Work out the finished part from the listing and answer in its coordinate system (mm). A direction names the side the tool comes from. Coordinates: 2 decimals unless noted, no trailing zeros. Order: outer loops, then holes, each group sorted by start corner. A loop starts at its lowest first (then second) coordinate and runs counter-clockwise, first axis right, second up. Notation, with made-up numbers: (46, -37.75) - (85, -37.75) arc R27 ccw to (85, -12.75) - close; hole circle Ø9 at (75, -19.5). An arc over 180 degrees is marked (long way). Use CSV: the item, a comma, the result in double quotes. Start each with the question number.
from build123d import *

# Parameters (mm, degrees)
SKETCH1_W           = 12
SKETCH1_H           = 10
BOSS_EXTRUDE1_DEPTH = 24.2
SKETCH2_R           = 1.5
BOSS_EXTRUDE2_DEPTH = 10
SKETCH3_R           = 0.65
CUT_EXTRUDE1_DEPTH  = 1


with BuildPart() as part:
    # Sketch1 → Boss-Extrude1 (new body)
    with BuildSketch(Plane(origin=(0, 0, 0), x_dir=(0, 0, -1), z_dir=(1, 0, 0))):
        Rectangle(SKETCH1_W, SKETCH1_H)
    extrude(amount=BOSS_EXTRUDE1_DEPTH)

    # Sketch2 → Boss-Extrude2 (add)
    with BuildSketch(Plane(origin=(24.2, 0, 0), x_dir=(0, 0, -1), z_dir=(1, 0, 0))):
        Circle(SKETCH2_R)
    extrude(amount=BOSS_EXTRUDE2_DEPTH)

    # Sketch3 → Cut-Extrude1 (cut)
    with BuildSketch(Plane(origin=(24.2, 0, 0), x_dir=(0, 0, -1), z_dir=(1, 0, 0))):
        with Locations((-4.5, 0)):
            Circle(SKETCH3_R)
        with Locations((4.5, 0)):
            Circle(SKETCH3_R)
    extrude(amount=-CUT_EXTRUDE1_DEPTH, mode=Mode.SUBTRACT)


solid = part.part
1) Straight lines are drawn through the part: line 1 (Y direction, x = 23.85, z = -4.5); line 2 (X direction, y = 4.25, z = 3.25). For each, find the intervals that lie inside material, in ascending order. Write a range as [from, to].
2) For faces 1 (the face through (23.71, 0.2, 3.88)), 2 (the face through (12, 0, -6)), determine the directions among +Z, -Z, +X, -X, +Y, -Y from which every point of the face is accessible in a straight line to the end or side of a thin tool.
3) The part is cut by section D-D on y = -3.5. Determine the outline of the cut face in (x, z), plus the area to 3 significant figures.
4) The part is cut by section B-B on y = 0. Determine the outline of the cut face in (x, z).
5) Flat-ended cylindrical pins translate along their axes: P1, Ø2, axis at y = 0, z = -4.5, coming from the +X side; P2, Ø5, axis at y = 1, z = 2, coming from the +X side. Find the tip coordinate at first contact, or state that the pin passes through.
6) The part is cut by section C-C on z = -4.5. Determine the outline of the cut face in (x, y), plus the area to 3 significant figures.
7) For a pull along Z with two mould halves and no side action, classify faces 3 (the face through (0, 0, 0)), 4 (the face through (29.13, 0.07, 1.5)), 5 (the face through (23.71, 0.2, -5.12)), 6 (the face through (23.2, 0, 5)) as +Z half, -Z half, draft (parallel to the pull), parting line (faces both ways), or undercut.
8) The part is cut by section A-A on z = 0. Determine the outline of the cut face in (x, y), plus the area to 3 significant figures.
Answer key:
1,line 1,"[-5, -0.65], [0.65, 5]"
1,line 2,"[0, 24.2]"
2,face 1,"+X"
2,face 2,"-Z, +X, -X, +Y, -Y"
3,outline,"(0, -6) - (24.2, -6) - (24.2, 6) - (0, 6) - close"
3,area,"290 mm^2"
4,outline,"(0, -6) - (24.2, -6) - (24.2, -5.15) - (23.2, -5.15) - (23.2, -3.85) - (24.2, -3.85) - (24.2, -1.5) - (34.2, -1.5) - (34.2, 1.5) - (24.2, 1.5) - (24.2, 3.85) - (23.2, 3.85) - (23.2, 5.15) - (24.2, 5.15) - (24.2, 6) - (0, 6) - close"
5,P1,"x = 24.2"
5,P2,"x = 34.2"
6,outline,"(0, -5) - (24.2, -5) - (24.2, -0.65) - (23.2, -0.65) - (23.2, 0.65) - (24.2, 0.65) - (24.2, 5) - (0, 5) - close"
6,area,"241 mm^2"
7,face 3,"draft"
7,face 4,"parting line"
7,face 5,"undercut"
7,face 6,"undercut"
8,outline,"(0, -5) - (24.2, -5) - (24.2, -1.5) - (34.2, -1.5) - (34.2, 1.5) - (24.2, 1.5) - (24.2, 5) - (0, 5) - close"
8,area,"272 mm^2"
